Part model, mm, in its own coordinate system. A direction names the side the tool comes from. Round coordinates to 2 decimals unless told otherwise and drop trailing zeros. Loops run counter-clockwise (first coordinate to the right, second up) from the corner with the lowest first, then second, coordinate; pieces in that order, holes last. Notation, with made-up numbers: (-28.75, 65.25) - (-5.75, 65.25) arc R21 cw to (-5.75, 77.25) - close; hole circle Ø7 at (0, 43.5). An arc over 180 degrees is marked (long way). Put each result on its own line as item: value.
from build123d import *

# Parameters (mm, degrees)
SKETCH_R     = 2
PAD_DEPTH    = 15.1
SKETCH001_R  = 3.2
PAD001_DEPTH = 3
SKETCH002_R  = 1.25
PAD002_DEPTH = 3.4
SKETCH003_R  = 2
PAD003_DEPTH = 3
FILLET_R     = 0.5
FILLET001_R  = 0.5
FILLET002_R  = 0.5
FILLET003_R  = 1
FILLET004_R  = 1


with BuildPart() as part:
    # Sketch → Pad (new body)
    with BuildSketch(Plane.YZ):
        Circle(SKETCH_R)
    extrude(amount=PAD_DEPTH)

    # Sketch001 → Pad001 (join)
    with BuildSketch(Plane(origin=(0, 0, 0), x_dir=(0, 1, 0), z_dir=(-1, 0, 0))):
        Circle(SKETCH001_R)
    extrude(amount=PAD001_DEPTH)

    # Sketch002 → Pad002 (join)
    with BuildSketch(Plane.YZ.offset(15.1)):
        Circle(SKETCH002_R)
    extrude(amount=PAD002_DEPTH)

    # Sketch003 → Pad003 (join)
    with BuildSketch(Plane.YZ.offset(18.5)):
        Circle(SKETCH003_R)
    extrude(amount=PAD003_DEPTH)

    # Fillet
    fillet_edges = [part.edges().sort_by_distance(p)[0] for p in [
        (18.5, -2, 0),
    ]]
    fillet(fillet_edges, radius=FILLET_R)

    # Fillet001
    fillet001_edges = [part.edges().sort_by_distance(p)[0] for p in [
        (21.5, -2, 0),
    ]]
    fillet(fillet001_edges, radius=FILLET001_R)

    # Fillet002
    fillet002_edges = [part.edges().sort_by_distance(p)[0] for p in [
        (15.1, -2, 0),
    ]]
    fillet(fillet002_edges, radius=FILLET002_R)

    # Fillet003
    fillet003_edges = [part.edges().sort_by_distance(p)[0] for p in [
        (-3, -3.2, 0),
    ]]
    fillet(fillet003_edges, radius=FILLET003_R)

    # Fillet004
    fillet004_edges = [part.edges().sort_by_distance(p)[0] for p in [
        (0, -3.2, 0),
    ]]
    fillet(fillet004_edges, radius=FILLET004_R)


solid = part.part
1. Band-saw the part on C-C (x = 11.5). List the corners of the cut face in (y, z).
A:
outline: circle Ø4 at (0, 0)
2. Pin check, flat tips, straight feed: P1, Ø1.5, axis at x = 11, y = -0.5, coming from the -Z side; P2, Ø1.5, axis at x = 14, y = -2, coming from the -Z side; P3, Ø1, axis at x = 14, y = 1.5, coming from the +Z side. Stop position of each tip, or through.
A:
P1: stops at z = -2
P2: stops at z = -1.56
P3: stops at z = 1.73
3. Probe line 1 along X through (y, z) = (-2.25, 0); line 2 along Z through (x, y) = (1, 0); line 3 along X through (y, z) = (-1.5, 1). List the from-to ranges inside material, lowest first. Write a range as [from, to].
A:
line 1: x = [-3, 0]
line 2: z = [-2, 2]
line 3: x = [-3, 15], [18.6, 21.4]
4. Tool access for faces 1 (the cylindrical face through (16.78, -0.27, -1.22)), 2 (the flat face through (-3, 0, 0)), 3 (the cylindrical face through (20, 0, -2)): list every direction of +Z, -Z, +X, -X, +Y, -Y with a clear straight run to the whole face (end or side of a thin tool).
A:
face 1: none
face 2: +Z, -Z, -X, +Y, -Y
face 3: +X
5. Band-saw the part on D-D (x = 18). List the corners of the cut face in (y, z).
A:
outline: circle Ø2.5 at (0, 0)
6. Band-saw the part on A-A (z = 0). List the corners of the cut face in (x, y), plus the area to 3 significant figures.
A:
outline: (-3, -2.2) arc R1 ccw to (-2, -3.2) - (-1, -3.2) arc R1 ccw to (0, -2.2) - (0, -2) - (14.6, -2) arc R0.5 ccw to (15.1, -1.5) - (15.1, -1.25) - (18.5, -1.25) - (18.5, -1.5) arc R0.5 ccw to (19, -2) - (21, -2) arc R0.5 ccw to (21.5, -1.5) - (21.5, 1.5) arc R0.5 ccw to (21, 2) - (19, 2) arc R0.5 ccw to (18.5, 1.5) - (18.5, 1.25) - (15.1, 1.25) - (15.1, 1.5) arc R0.5 ccw to (14.6, 2) - (0, 2) - (0, 2.2) arc R1 ccw to (-1, 3.2) - (-2, 3.2) arc R1 ccw to (-3, 2.2) - close
area: 98.9 mm²
